Input: dimensioned drawing with shaded views. Units: mm. Origin: part minimum x, y, z. Coordinates: 2 decimals unless noted, no trailing zeros. Loops run counter-clockwise (first coordinate to the right, second up) from the corner with the lowest first, then second, coordinate; pieces in that order, holes last.
Item 1: Pin query (flat end, axial travel): pin 1 Ø5.5 at (y, z) = (10.5, 387.5) entering from +X; pin 2 Ø5.5 at (y, z) = (8, 150) entering from -X; pin 3 Ø9.5 at (x, y) = (71.5, 11) entering from -Z. Return the tip coordinate at first contact, or that it passes through.
Item 2: Section query A-A, the plane x = 243. Return the cut outline in (y, z).
Item 3: Line query: probe 1 along X at (y, z) = (1, 243); probe 2 along X at (y, z) = (6.75, 333.5). Output: solid intervals per line, ascending.
Item 4: Section query B-B, the plane z = 204.5. Return the cut outline in (x, y).
Item 5: Section query D-D, the plane x = 89. Return the cut outline in (y, z).
Item 6: Section query C-C, the plane y = 16. Return the cut outline in (x, z).
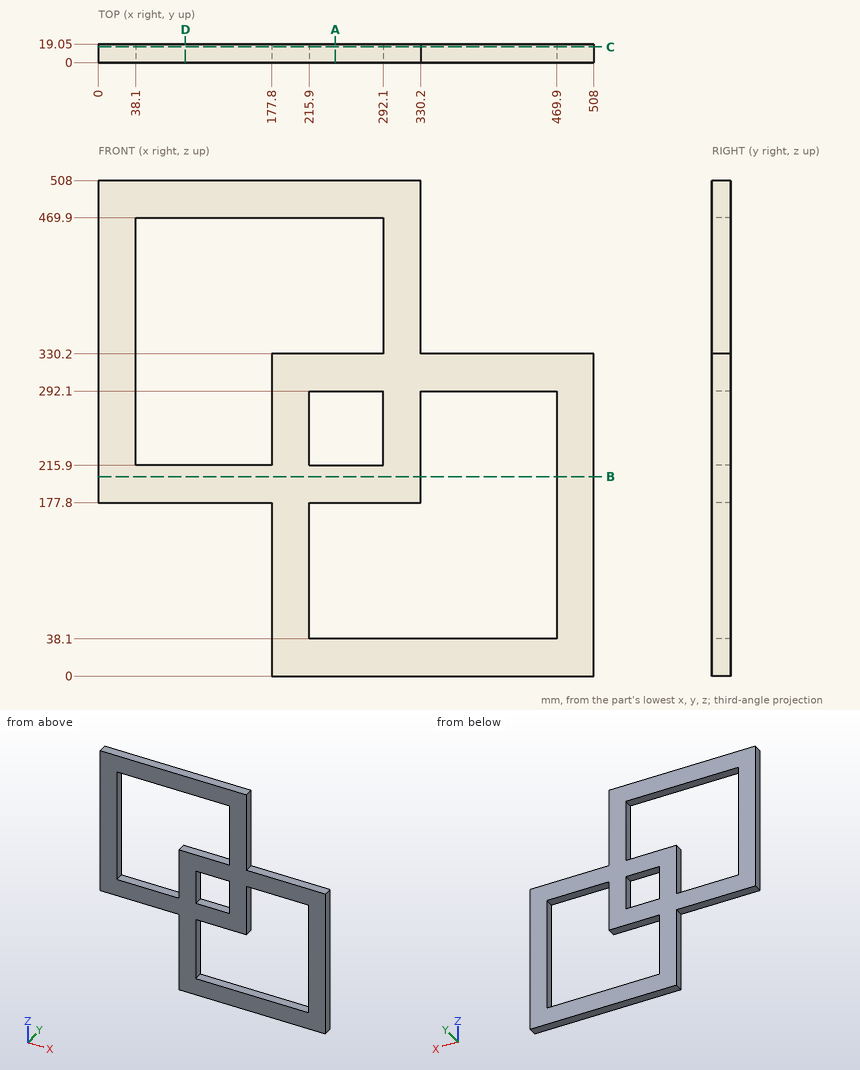
Verdict:
1. pin 1: stops at x = 330.2
1. pin 2: stops at x = 177.8
1. pin 3: stops at z = 177.8
2. outline: (0, 0) - (19.05, 0) - (19.05, 38.1) - (0, 38.1) - close; (0, 177.8) - (19.05, 177.8) - (19.05, 215.9) - (0, 215.9) - close; (0, 292.1) - (19.05, 292.1) - (19.05, 330.2) - (0, 330.2) - close; (0, 469.9) - (19.05, 469.9) - (19.05, 508) - (0, 508) - close
3. probe 1: x = 0 to 38.1, 177.8 to 215.9, 292.1 to 330.2, 469.9 to 508
3. probe 2: x = 0 to 38.1, 292.1 to 330.2
4. outline: (0, 0) - (330.2, 0) - (330.2, 19.05) - (0, 19.05) - close; (469.9, 0) - (508, 0) - (508, 19.05) - (469.9, 19.05) - close
5. outline: (0, 177.8) - (19.05, 177.8) - (19.05, 215.9) - (0, 215.9) - close; (0, 469.9) - (19.05, 469.9) - (19.05, 508) - (0, 508) - close
6. outline: (0, 177.8) - (177.8, 177.8) - (177.8, 0) - (508, 0) - (508, 330.2) - (330.2, 330.2) - (330.2, 508) - (0, 508) - close; hole (38.1, 215.9) - (177.8, 215.9) - (177.8, 330.2) - (292.1, 330.2) - (292.1, 469.9) - (38.1, 469.9) - close; hole (215.9, 38.1) - (469.9, 38.1) - (469.9, 292.1) - (330.2, 292.1) - (330.2, 177.8) - (215.9, 177.8) - close; hole (215.9, 215.9) - (292.1, 215.9) - (292.1, 292.1) - (215.9, 292.1) - close
